Verification items for this drawing (mm, ordinates from the low corner). Round coordinates to 2 decimals unless told otherwise and drop trailing zeros. Loops run counter-clockwise (first coordinate to the right, second up) from the corner with the lowest first, then second, coordinate; pieces in that order, holes last. Notation, with made-up numbers: (-22, 66.25) - (9, 66.25) arc R28 cw to (9, 98.25) - close; hole circle Ø4 at (3, 46.5). An arc over 180 degrees is marked (long way). Answer in a Markdown table with one row per item. Add a question column.
(1) Cross-section at C-C on y = 127. Enter the section's corners in (x, z).
(2) Thickness scan on line 1 along X through (y, z) = (107.95, 7.5); line 2 along Y through (x, z) = (104.5, 159.5). Record the ranges inside material, lowest first.
(3) Cross-section at A-A on z = 254. Enter the section's corners in (x, y), then the cut area to 3 significant figures.
(4) Cross-section at D-D on z = 150. Enter the section's corners in (x, y).
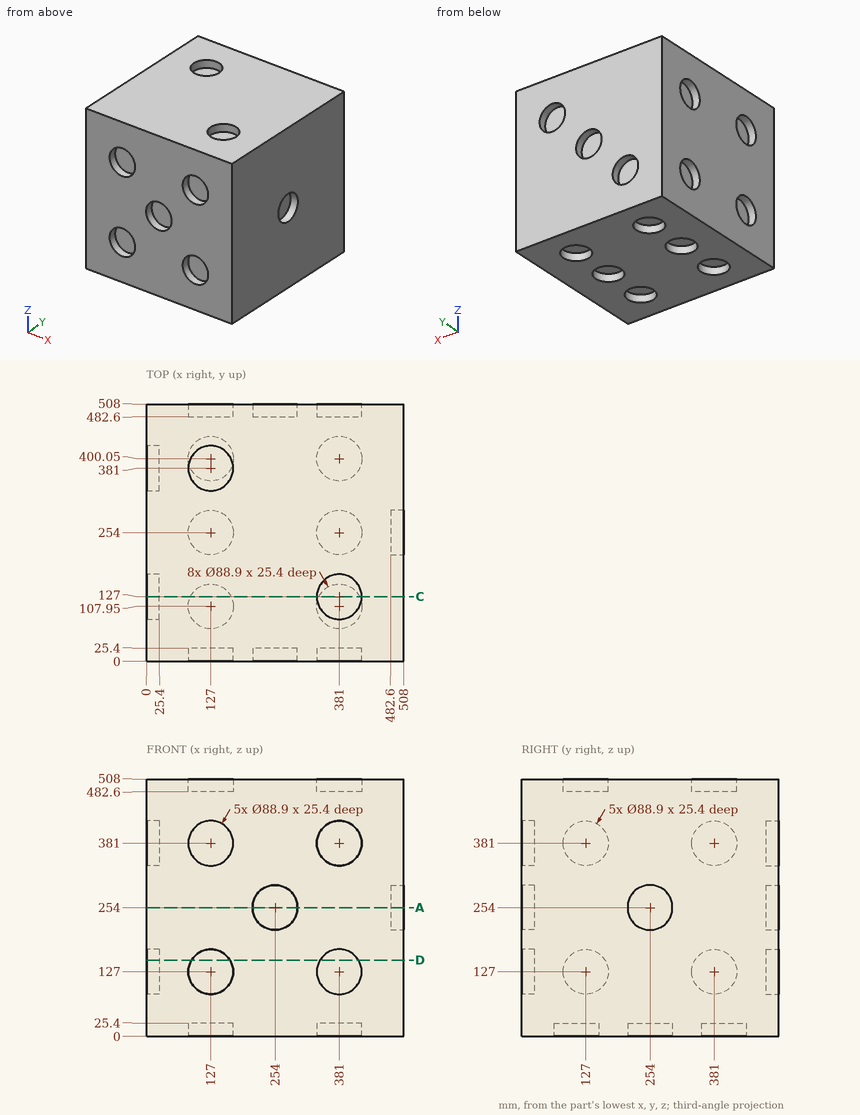
Answers:
| question | item | result |
|---|---|---|
| 1 | outline | (0, 0) - (86.84, 0) - (86.84, 25.4) - (167.16, 25.4) - (167.16, 0) - (340.84, 0) - (340.84, 25.4) - (421.16, 25.4) - (421.16, 0) - (508, 0) - (508, 508) - (425.45, 508) - (425.45, 482.6) - (336.55, 482.6) - (336.55, 508) - (0, 508) - (0, 425.45) - (25.4, 425.45) - (25.4, 336.55) - (0, 336.55) - (0, 171.45) - (25.4, 171.45) - (25.4, 82.55) - (0, 82.55) - close |
| 2 | line 1 | x = 0 to 82.55, 171.45 to 336.55, 425.45 to 508 |
| 2 | line 2 | y = 25.4 to 482.6 |
| 3 | outline | (0, 0) - (209.55, 0) - (209.55, 25.4) - (298.45, 25.4) - (298.45, 0) - (508, 0) - (508, 209.55) - (482.6, 209.55) - (482.6, 298.45) - (508, 298.45) - (508, 508) - (298.45, 508) - (298.45, 482.6) - (209.55, 482.6) - (209.55, 508) - (0, 508) - close |
| 3 | area | 251,000 mm^2 |
| 4 | outline | (0, 0) - (88.96, 0) - (88.96, 25.4) - (165.04, 25.4) - (165.04, 0) - (342.96, 0) - (342.96, 25.4) - (419.04, 25.4) - (419.04, 0) - (508, 0) - (508, 508) - (165.04, 508) - (165.04, 482.6) - (88.96, 482.6) - (88.96, 508) - (0, 508) - (0, 419.04) - (25.4, 419.04) - (25.4, 342.96) - (0, 342.96) - (0, 165.04) - (25.4, 165.04) - (25.4, 88.96) - (0, 88.96) - close |
